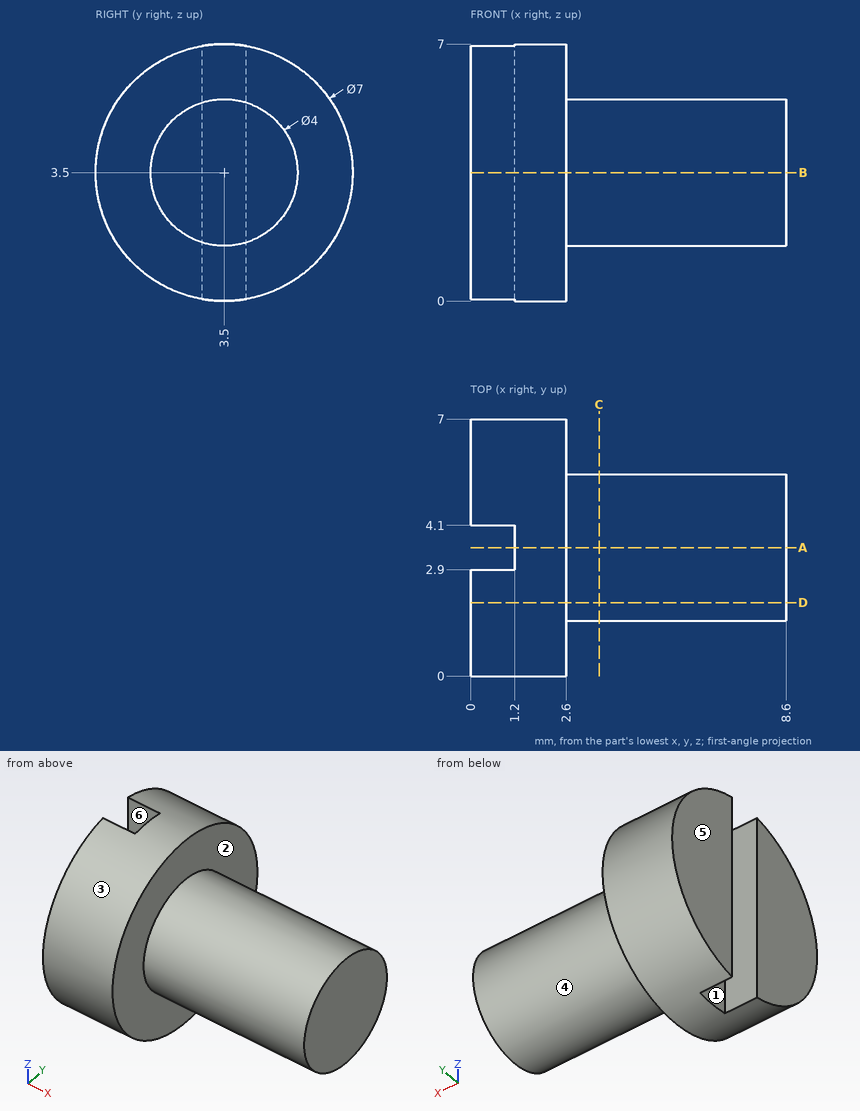
Here's the drawing with two shaded views (mm, measured from the low corner). I have some questions. A direction names the side the tool comes from. Give positions to 0.01 mm unless a question says otherwise; leave off trailing zeros. Order: outer loops, then holes, each group sorted by start corner. A loop starts at its lowest first (then second) coordinate and runs counter-clockwise, first axis right, second up. Notation, with made-up numbers: M 27.25,-16.5 L 79.25,-16.5 A29 cw 79.25,4.5 Z; hole C -31,42.25 d6. An arc over 180 degrees is marked long. Answer as a JSON object with one key per item and string values. Group by question number.
1) I'm going to push flat-ended pins straight in: pin 1 Ø1 at (x, z) = (1, 2) entering from -Y; pin 2 Ø4 at (x, y) = (5.5, 4.5) entering from +Z; pin 3 Ø1 at (x, z) = (7, 2.5) entering from +Y. Where does each tip first touch, or does it pass through?
2) We'd pull the mould along Y, two halves only. Please class the marked faces 4, 5 and 6: pulls with the +Y half, pulls with the -Y half, needs draft (parallel to the pull), parting line crosses it, or undercut.
3) Suppose I cut it at D-D, the plane y = 2. Write out the boundary of the cut face in (x, z), plus the area to 3 significant figures.
4) On a 3-axis mill with a long thin cutter (end or side, diameter ignored), from which of +Z, -Z, +X, -X, +Y, -Y can I reach the whole of each face in a straight line? I mean the marked faces 1, 2 and 3. Say none if no direction works.
5) Please list where these lines run through material, in increasing order: L1, parallel to X at y = 5.75, z = 4.5; L2, parallel to Y at x = 5.5, z = 3.5; L3, parallel to X at y = 3.75, z = 3. Write a range as [from, to].
6) Suppose I cut it at C-C, the plane x = 3.5. Write out the boundary of the cut face in (y, z).
7) Suppose I cut it at A-A, the plane y = 3.5. Write out the boundary of the cut face in (x, z), plus the area to 3 significant figures.
8) Suppose I cut it at B-B, the plane z = 3.5. Write out the boundary of the cut face in (x, y).
Results found:
{
 "1": {"pin 1": "y = 0.15", "pin 2": "z = 5.5", "pin 3": "y = 5.44"},
 "2": {"face 4": "parting line crosses it", "face 5": "needs draft", "face 6": "undercut"},
 "3": {"outline": "M 0,0.34 L 2.6,0.34 L 2.6,2.18 L 8.6,2.18 L 8.6,4.82 L 2.6,4.82 L 2.6,6.66 L 0,6.66 Z", "area": "32.3 mm²"},
 "4": {"face 1": "+Z, -Z, -X", "face 2": "+X", "face 3": "+X, -X"},
 "5": {"L1": "[0, 2.6]", "L2": "[1.5, 5.5]", "L3": "[1.2, 8.6]"},
 "6": {"outline": "C 3.5,3.5 d4"},
 "7": {"outline": "M 1.2,0 L 2.6,0 L 2.6,1.5 L 8.6,1.5 L 8.6,5.5 L 2.6,5.5 L 2.6,7 L 1.2,7 Z", "area": "33.8 mm²"},
 "8": {"outline": "M 0,0 L 2.6,0 L 2.6,1.5 L 8.6,1.5 L 8.6,5.5 L 2.6,5.5 L 2.6,7 L 0,7 L 0,4.1 L 1.2,4.1 L 1.2,2.9 L 0,2.9 Z"}
}
